Job drawing, mm, ordinate dimensions from the low corner. One solid piece. A direction names the side the tool comes from. Give positions to 0.01 mm unless a question says otherwise; leave off trailing zeros. Loops run counter-clockwise (first coordinate to the right, second up) from the corner with the lowest first, then second, coordinate; pieces in that order, holes last. Notation, with made-up numbers: M 42,50 L 87,50 A10 cw 87,65 Z; hole C 50,-30 d4. An arc over 180 degrees is marked long. One line per question, with ' | ' between items.
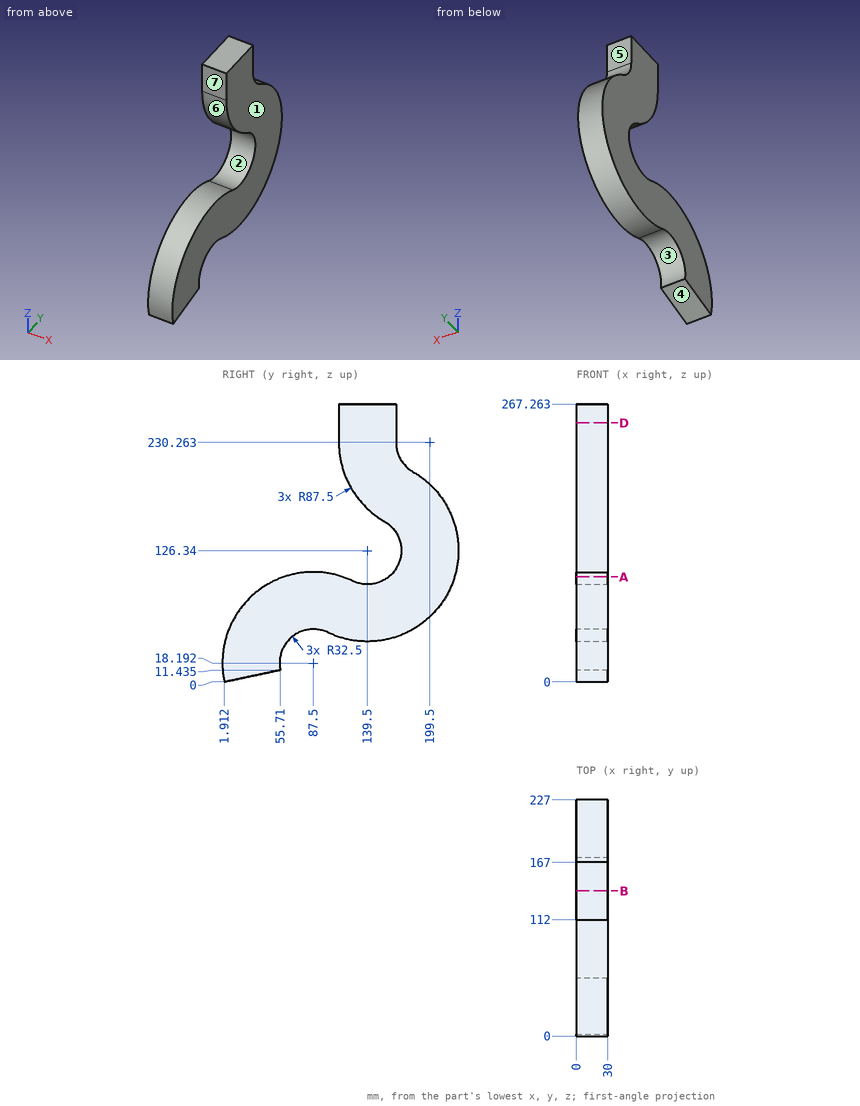
Item 1: Mould opens along Z. For the marked faces 1, 2, 3 and 4 say: pulls with the +Z half, pulls with the -Z half, needs draft (parallel to the pull), parting line crosses it, or undercut.
Conclusion:
face 1: needs draft | face 2: undercut | face 3: undercut | face 4: pulls with the -Z half
Item 2: Drill centre lines: line 1 along Z through (x, y) = (16.5, 129.5) (1 decimal); line 2 along Y through (x, z) = (19, 126.5); line 3 along Z through (x, y) = (22.75, 121) (1 decimal). Where is each one in solid material? Low to high. Write a range as [from, to].
Conclusion:
line 1: [39.4, 95.4], [177.8, 267.3] | line 2: [172, 227] | line 3: [40.8, 99], [191.6, 267.3]
Item 3: Drop flat-ended pins along their axis: P1, Ø15, axis at x = 14.5, z = 253.5, coming from the -Y side; P2, Ø5, axis at x = 24.5, z = 67.5, coming from the +Y side; P3, Ø6, axis at x = 24.5, z = 221, coming from the +Y side. Give the stop position or say it passes through.
Conclusion:
P1: y = 112 | P2: y = 206.45 | P3: y = 169.4
Item 4: Saw through at D-D on z = 249. Give the cut face in (x, y).
Conclusion:
outline: M 0,112 L 30,112 L 30,167 L 0,167 Z
Item 5: 3-axis set-ups, long thin cutter, end or side, ignore diameter. For the marked faces 5, 6 and 7: which of +Z, -Z, +X, -X, +Y, -Y reach the whole face in a straight line?
Conclusion:
face 5: +Z, +X, -X, +Y | face 6: +X, -X, -Y | face 7: +Z, +X, -X, -Y
Item 6: Saw through at A-A on z = 101. Give the cut face in (x, y), and give its area (3 significant figures).
Conclusion:
outline: M 0,59.23 L 30,59.23 L 30,115.77 L 0,115.77 Z; M 0,159.85 L 30,159.85 L 30,223.25 L 0,223.25 Z | area: 3,600 mm²
Item 7: Saw through at B-B on y = 139.5. Give the cut face in (x, z) (1 decimal), and give its area (3 significant figures).
Conclusion:
outline: M 0,38.8 L 30,38.8 L 30,93.8 L 0,93.8 Z; M 0,166.6 L 30,166.6 L 30,267.3 L 0,267.3 Z | area: 4,670 mm²
